Verification items for the finished model (mm, model axes). Face numbers are marked on the shaded views. A direction names the side the tool comes from. Coordinates: 2 decimals unless noted, no trailing zeros. Order: outer loops, then holes, each group sorted by start corner. A loop starts at its lowest first (then second) coordinate and runs counter-clockwise, first axis right, second up. Notation, with made-up numbers: M -1,-12.5 L 39,-12.5 A12 cw 39,0.5 Z; hole C -5.5,-21 d11. An arc over 180 degrees is marked long. Use one line per item in the form item = value. Start each with the question number.
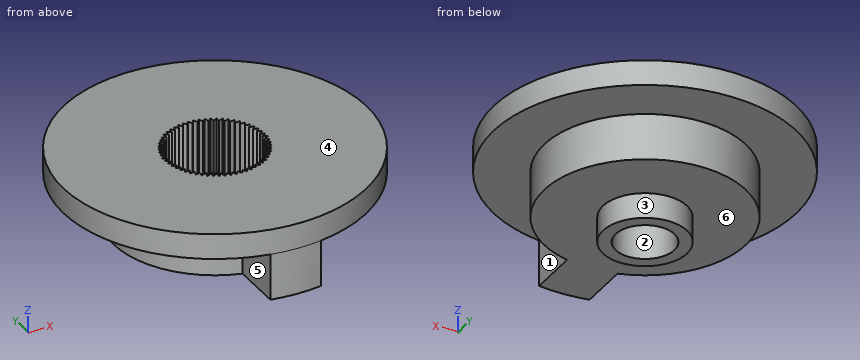
```python
from build123d import *

# Parameters (mm, degrees)
BASE_EXTRUSION_DEPTH    = 2.75
ESQUISSE3_R             = 9
BOSS_EXTRU_1_DEPTH      = 1.5
ENL_V_MAT_EXTRU_2_DEPTH = 5.25
ESQUISSE5_R             = 4
BOSS_EXTRU_2_DEPTH      = 1
ESQUISSE6_R             = 2.5
BOSS_EXTRU_3_DEPTH      = 1.5
ESQUISSE7_R             = 1.75
ENL_V_MAT_EXTRU_3_DEPTH = 6.75


with BuildPart() as part:
    # Esquisse2 → Base-Extrusion (new body)
    with BuildSketch(Plane.XY):
        with BuildLine():
            Line((1.5, -5.809475019), (1.5, -8.874119675))
            ThreePointArc((1.5, -8.874119675), (0, -9), (-1.5, -8.874119675))
            Line((-1.5, -8.874119675), (-1.5, -5.809475019))
            ThreePointArc((-1.5, -5.809475019), (0, 6), (1.5, -5.809475019))
        make_face()
    extrude(amount=BASE_EXTRUSION_DEPTH)

    # Esquisse3 → Boss.-Extru.1 (add)
    with BuildSketch(Plane.XY.offset(2.75)):
        Circle(ESQUISSE3_R)
    extrude(amount=BOSS_EXTRU_1_DEPTH)

    # Esquisse1 → Enlèv. mat.-Extru.2 (cut, through all)
    with BuildSketch(Plane.XY):
        Polygon((0, 3), (-0.14392388, 2.746231221), (-0.31358539, 2.983565686), (-0.430194779, 2.716142937), (-0.623735072, 2.934442802), (-0.711752374, 2.656296022), (-0.927050983, 2.853169549), (-0.985511861, 2.567346173), (-1.220209929, 2.740636373), (-1.248473874, 2.450267942), (-1.5, 2.598076211), (-1.497757346, 2.306344062), (-1.763355757, 2.427050983), (-1.730631075, 2.137151394), (-2.007391819, 2.229434476), (-1.944543648, 1.944543648), (-2.229434476, 2.007391819), (-2.137151394, 1.730631075), (-2.427050983, 1.763355757), (-2.306344062, 1.497757346), (-2.598076211, 1.5), (-2.450267942, 1.248473874), (-2.740636373, 1.220209929), (-2.567346173, 0.985511861), (-2.853169549, 0.927050983), (-2.656296022, 0.711752374), (-2.934442802, 0.623735072), (-2.716142937, 0.430194779), (-2.983565686, 0.31358539), (-2.746231221, 0.14392388), (-3, 0), (-2.746231221, -0.14392388), (-2.983565686, -0.31358539), (-2.716142937, -0.430194779), (-2.934442802, -0.623735072), (-2.656296022, -0.711752374), (-2.853169549, -0.927050983), (-2.567346173, -0.985511861), (-2.740636373, -1.220209929), (-2.450267942, -1.248473874), (-2.598076211, -1.5), (-2.306344062, -1.497757346), (-2.427050983, -1.763355757), (-2.137151394, -1.730631075), (-2.229434476, -2.007391819), (-1.944543648, -1.944543648), (-2.007391819, -2.229434476), (-1.730631075, -2.137151394), (-1.763355757, -2.427050983), (-1.497757346, -2.306344062), (-1.5, -2.598076211), (-1.248473874, -2.450267942), (-1.220209929, -2.740636373), (-0.985511861, -2.567346173), (-0.927050983, -2.853169549), (-0.711752374, -2.656296022), (-0.623735072, -2.934442802), (-0.430194779, -2.716142937), (-0.31358539, -2.983565686), (-0.14392388, -2.746231221), (0, -3), (0.14392388, -2.746231221), (0.31358539, -2.983565686), (0.430194779, -2.716142937), (0.623735072, -2.934442802), (0.711752374, -2.656296022), (0.927050983, -2.853169549), (0.985511861, -2.567346173), (1.220209929, -2.740636373), (1.248473874, -2.450267942), (1.5, -2.598076211), (1.497757346, -2.306344062), (1.763355757, -2.427050983), (1.730631075, -2.137151394), (2.007391819, -2.229434476), (1.944543648, -1.944543648), (2.229434476, -2.007391819), (2.137151394, -1.730631075), (2.427050983, -1.763355757), (2.306344062, -1.497757346), (2.598076211, -1.5), (2.450267942, -1.248473874), (2.740636373, -1.220209929), (2.567346173, -0.985511861), (2.853169549, -0.927050983), (2.656296022, -0.711752374), (2.934442802, -0.623735072), (2.716142937, -0.430194779), (2.983565686, -0.31358539), (2.746231221, -0.14392388), (3, 0), (2.746231221, 0.14392388), (2.983565686, 0.31358539), (2.716142937, 0.430194779), (2.934442802, 0.623735072), (2.656296022, 0.711752374), (2.853169549, 0.927050983), (2.567346173, 0.985511861), (2.740636373, 1.220209929), (2.450267942, 1.248473874), (2.598076211, 1.5), (2.306344062, 1.497757346), (2.427050983, 1.763355757), (2.137151394, 1.730631075), (2.229434476, 2.007391819), (1.944543648, 1.944543648), (2.007391819, 2.229434476), (1.730631075, 2.137151394), (1.763355757, 2.427050983), (1.497757346, 2.306344062), (1.5, 2.598076211), (1.248473874, 2.450267942), (1.220209929, 2.740636373), (0.985511861, 2.567346173), (0.927050983, 2.853169549), (0.711752374, 2.656296022), (0.623735072, 2.934442802), (0.430194779, 2.716142937), (0.31358539, 2.983565686), (0.14392388, 2.746231221), align=None)
    extrude(amount=ENL_V_MAT_EXTRU_2_DEPTH, mode=Mode.SUBTRACT)

    # Esquisse5 → Boss.-Extru.2 (add)
    with BuildSketch(Plane(origin=(0, 0, 0), x_dir=(-1, 0, 0), z_dir=(0, 0, -1))):
        Circle(ESQUISSE5_R)
    extrude(amount=-BOSS_EXTRU_2_DEPTH)

    # Esquisse6 → Boss.-Extru.3 (add)
    with BuildSketch(Plane(origin=(0, 0, 0), x_dir=(-1, 0, 0), z_dir=(0, 0, -1))):
        Circle(ESQUISSE6_R)
    extrude(amount=BOSS_EXTRU_3_DEPTH)

    # Esquisse7 → Enlèv. mat.-Extru.3 (cut, through all)
    with BuildSketch(Plane(origin=(0, 0, -1.5), x_dir=(-1, 0, 0), z_dir=(0, 0, -1))):
        Circle(ESQUISSE7_R)
    extrude(amount=-ENL_V_MAT_EXTRU_3_DEPTH, mode=Mode.SUBTRACT)


solid = part.part
```
1. Release check for a two-part mould opening along Y. For the marked faces 1, 2 and 3 record: pulls with the +Y half, pulls with the -Y half, needs draft (parallel to the pull), parting line crosses it, or undercut.
2. Cross-section at C-C on y = 7.75. Enter the section's corners in (x, z), and give its area (3 significant figures).
3. Material ranges on line 1 along Y through (x, z) = (0, -0.8); line 2 along Y through (x, z) = (0, 0.45); line 3 along Z through (x, y) = (2, 6.5), recorded low to high.
4. Tool access check on the marked faces 4, 5 and 6. Record the directions out of +Z, -Z, +X, -X, +Y, -Y that give a thin tool (end or side, any length) a straight path to the whole face; none if there is none.
5. Depth check by flat-ended pin: P1, Ø1.4, axis at y = -8, z = 1, coming from the -X side; P2, Ø1, axis at y = 2.5, z = 2, coming from the +X side; P3, Ø3, axis at x = 0, y = 0, coming from the -Z side; P4, Ø1.5, axis at x = 4, z = -0.5, coming from the +Y side. Enter the tip coordinate at first touch or a pass-through.
6. Cross-section at B-B on y = -6.5. Enter the section's corners in (x, z), and give its area (3 significant figures).
7. Cross-section at A-A on x = 5.25. Enter the section's corners in (y, z), and give its area (3 significant figures).
Final values:
q1.face_1 = needs draft
q1.face_2 = undercut
q1.face_3 = parting line crosses it
q2.outline = M -4.58,2.75 L 4.58,2.75 L 4.58,4.25 L -4.58,4.25 Z
q2.area = 13.7 mm2
q3.line_1 = -2.5 to -1.75, 1.75 to 2.5
q3.line_2 = -9 to -1.75, 1.75 to 6
q3.line_3 = 2.75 to 4.25
q4.face_4 = +Z, +X, -X, +Y, -Y
q4.face_5 = -Z, -X, -Y
q4.face_6 = -Z
q5.P1 = -1.5
q5.P2 = 5.66
q5.P3 = through
q5.P4 = 4.92
q6.outline = M -6.22,2.75 L -1.5,2.75 L -1.5,0 L 1.5,0 L 1.5,2.75 L 6.22,2.75 L 6.22,4.25 L -6.22,4.25 Z
q6.area = 26.9 mm2
q7.outline = M -7.31,2.75 L -2.9,2.75 L -2.9,0 L 2.9,0 L 2.9,2.75 L 7.31,2.75 L 7.31,4.25 L -7.31,4.25 Z
q7.area = 37.9 mm2
